For this review, take the finished solid that the model builds, in its own axes (mm). A direction names the side the tool comes from. Coordinates: 2 decimals unless noted, no trailing zeros. Loops run counter-clockwise (first coordinate to the right, second up) from the corner with the lowest first, then second, coordinate; pieces in that order, holes last. Notation, with made-up numbers: (-32.5, 65.5) -> (2.5, 65.5) arc R28 cw to (2.5, 98.5) -> close; hole circle Ø11 at (6, 26). An arc over 180 degrees is marked (long way). Use a Markdown table: item, result.
from build123d import *

# Parameters (mm, degrees)
SKETCH044_W     = 65
SKETCH044_H     = 35
PAD003_DEPTH    = 3
CHAMFER009_SIZE = 3
SKETCH054_W     = 2.32
SKETCH054_H     = 2.32
PAD004_DEPTH    = 6.2
FILLET_R        = 2
SKETCH055_R     = 1.4
POCKET007_DEPTH = 5


with BuildPart() as part:
    # Sketch044 → Pad003 (new body)
    with BuildSketch(Plane.XZ):
        with Locations((-0.83, 8.83)):
            Rectangle(SKETCH044_W, SKETCH044_H)
        Polygon((0, -1), (-27.85, -1), (-27.85, 7.89), (-21.74, 7.89), (-21.74, 10.21), (-27.85, 10.21), (-27.85, 17.05), (6.61, 17.05), (6.61, 14.52), (27.58, 14.52), (27.58, -1), align=None, mode=Mode.SUBTRACT)
    extrude(amount=PAD003_DEPTH)

    # Chamfer009
    chamfer009_edges = [part.edges().sort_by_distance(p)[0] for p in [
        (31.67, -1.5, 26.33),
        (31.67, -1.5, -8.67),
        (-33.33, -1.5, 26.33),
        (-33.33, -1.5, -8.67),
    ]]
    chamfer(chamfer009_edges, length=CHAMFER009_SIZE)

    # Sketch054 (on Face2 of Chamfer009) → Pad004 (join)
    with BuildSketch(Plane(origin=(0, 0, 0), x_dir=(1, 0, 0), z_dir=(0, 1, 0))):
        with Locations((-22.9, -9.05)):
            Rectangle(SKETCH054_W, SKETCH054_H)
    extrude(amount=PAD004_DEPTH)

    # Fillet
    fillet_edges = [part.edges().sort_by_distance(p)[0] for p in [
        (-27.85, -1.5, 17.05),
        (6.61, -1.5, 14.52),
        (27.58, -1.5, 14.52),
        (-27.85, -1.5, -1),
        (27.58, -1.5, -1),
        (-24.06, 0, 9.05),
    ]]
    fillet(fillet_edges, radius=FILLET_R)

    # Sketch055 (on Face26 of Fillet) → Pocket007 (cut)
    with BuildSketch(Plane.XZ.offset(3)):
        with Locations((-30.33, 23.33)):
            Circle(SKETCH055_R)
        with Locations((28.67, 23.33)):
            Circle(SKETCH055_R)
        with Locations((-30.33, -5.67)):
            Circle(SKETCH055_R)
        with Locations((28.67, -5.67)):
            Circle(SKETCH055_R)
    extrude(amount=-POCKET007_DEPTH, mode=Mode.SUBTRACT)


with BuildPart() as part_1:
    # Body013 placement: moved
    add(part.part.moved(Location((0, -51.5, 0))))


solid = part_1.part
(1) Take a section at B-B on z = 4.5. Write out the cut boundary in (x, y), plus the area to 3 significant figures.
Found:
| item | result |
|---|---|
| outline | (-33.33, -54.5) -> (-27.85, -54.5) -> (-27.85, -51.5) -> (-33.33, -51.5) -> close; (27.58, -54.5) -> (31.67, -54.5) -> (31.67, -51.5) -> (27.58, -51.5) -> close |
| area | 28.7 mm^2 |
(2) Take a section at A-A on x = 22. Write out the cut boundary in (y, z).
Found:
| item | result |
|---|---|
| outline | (-54.5, -8.67) -> (-51.5, -8.67) -> (-51.5, -1) -> (-54.5, -1) -> close; (-54.5, 14.52) -> (-51.5, 14.52) -> (-51.5, 26.33) -> (-54.5, 26.33) -> close |
(3) For faces 1 (the face through (-32, -53, -7)), 2 (the face through (-24.06, -47, 9)), 3 (the face through (-27.85, -53, 4)), list the 3-axis set-ups (+Z, -Z, +X, -X, +Y, -Y) from which the entire face can be reached by the end or side of a thin tool; tool diameter is ignored.
Found:
| item | result |
|---|---|
| face 1 | -Z, -X, +Y, -Y |
| face 2 | +Z, -Z, -X, +Y |
| face 3 | +Y, -Y |
(4) Take a section at C-C on y = -47.25. Write out the cut boundary in (x, z), plus the area to 3 significant figures.
Found:
| item | result |
|---|---|
| outline | (-24.06, 7.89) -> (-21.74, 7.89) -> (-21.74, 10.21) -> (-24.06, 10.21) -> close |
| area | 5.38 mm^2 |
(5) Mouldability with a two-part tool opening along X and no side actions: class faces 4 (the face through (-1, -53, 26.33)), 5 (the face through (-31.81, -52.98, 24.85)), 6 (the face through (-30.51, -53.02, 24.72)) as pulls with the +X half, pulls with the -X half, needs draft (parallel to the pull), parting line crosses it, or undercut.
Found:
| item | result |
|---|---|
| face 4 | needs draft |
| face 5 | pulls with the -X half |
| face 6 | undercut |
(6) For pin 1 Ø0.7 at (y, z) = (-47, 9) entering from -X; pin 2 Ø17.5 at (x, z) = (-13.5, 16) entering from +Y; pin 3 Ø1.8 at (x, y) = (-24.5, -49.5) entering from -Z, all flat-tipped, find the tip position at first contact; note any pin that passes through.
Found:
| item | result |
|---|---|
| pin 1 | stops at x = -24.06 |
| pin 2 | stops at y = -51.5 |
| pin 3 | stops at z = 7.89 |
(7) For line 1 along Z through (x, y) = (-30.33, -52.6); line 2 along X through (y, z) = (-51.75, 4); line 3 along Z through (x, y) = (-9.5, -51.75), list the stretches that pass through material, from the lowest coordinate up.
Found:
| item | result |
|---|---|
| line 1 | z = -8.67 to -7.07, -4.27 to 21.93, 24.73 to 26.33 |
| line 2 | x = -33.33 to -27.85, 27.58 to 31.67 |
| line 3 | z = -8.67 to -1, 17.05 to 26.33 |
